Check sheet for the modelled part. Datum: model origin and axes. Units: mm. Coordinates: 2 decimals unless noted, no trailing zeros. Loops run counter-clockwise (first coordinate to the right, second up) from the corner with the lowest first, then second, coordinate; pieces in that order, holes last. Notation, with made-up numbers: M 54,29 L 103,29 A19 cw 103,56 Z; hole C 54,-9.5 d2. An arc over 180 degrees is marked long. Use CSV: the item, a comma, the result in double quotes. Start each with the question number.
(1) Section check C-C on y = 1. Record the cut outline in (x, z), and give its area (3 significant figures).
(2) Go/stop test with flat-tipped pins: pin 1 Ø2 at (y, z) = (6.5, 11) entering from -X; pin 2 Ø4 at (x, y) = (-10, 3.5) entering from -Z. Record where each tip stops, or that it passes through.
(3) Section check D-D on y = 9.25. Record the cut outline in (x, z), and give its area (3 significant figures).
(4) Scan lines: line 1 (X direction, y = -0.5, z = 6); line 2 (X direction, y = 0.5, z = 11.25); line 3 (X direction, y = -11.75, z = 18.25). Record each from-to range of solid material in increasing order.
(5) Section check A-A on z = 14. Record the cut outline in (x, y), and give its area (3 significant figures).
(6) Section check B-B on y = -2.5. Record the cut outline in (x, z).
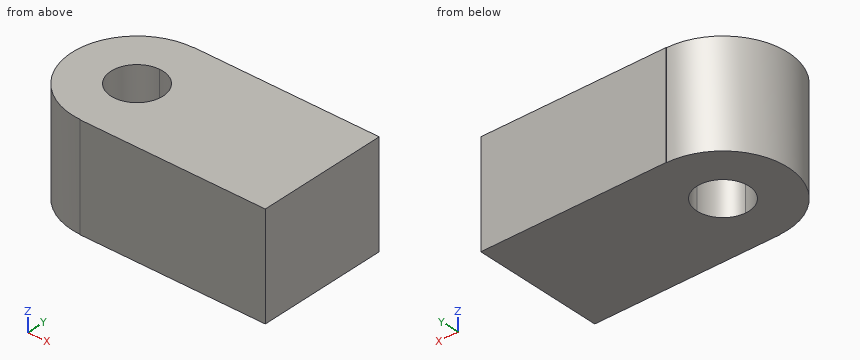
from build123d import *

# Parameters (mm, degrees)
F1_DEPTH = 20


with BuildPart() as f1:
    # F0 (on Top) → F1 (new body)
    with BuildSketch(Plane.XY):
        with BuildLine():
            Line((-12.4044854931, 4.3749214336), (-12.4044854931, 11.8749214336))
            ThreePointArc((-12.4044854931, 11.8749214336), (-24.9044854931, -0.6250785664), (-12.4044854931, -13.1250785664))
            Line((-12.4044854931, -13.1250785664), (-12.4044854931, -5.6250785664))
            ThreePointArc((-12.4044854931, -5.6250785664), (-17.4044854931, -0.6250785664), (-12.4044854931, 4.3749214336))
        make_face()
        with BuildLine():
            ThreePointArc((0.0955145069, -0.6250785664), (-3.5656507283, 8.2137561985), (-12.4044854931, 11.8749214336))
            Line((-12.4044854931, 11.8749214336), (-12.4044854931, 4.3749214336))
            ThreePointArc((-12.4044854931, 4.3749214336), (-8.8689515872, 2.9104553396), (-7.4044854931, -0.6250785664))
            ThreePointArc((-7.4044854931, -0.6250785664), (-8.8689515872, -4.1606124723), (-12.4044854931, -5.6250785664))
            Line((-12.4044854931, -5.6250785664), (-12.4044854931, -13.1250785664))
            ThreePointArc((-12.4044854931, -13.1250785664), (-3.5656507283, -9.4639133312), (0.0955145069, -0.6250785664))
        make_face()
        with BuildLine():
            Line((23.2241750516, 11.9398952645), (-12.4044854931, 11.9398952645))
            Line((-12.4044854931, 11.9398952645), (-12.4044854931, 11.8749214336))
            ThreePointArc((-12.4044854931, 11.8749214336), (-3.5656507283, 8.2137561985), (0.0955145069, -0.6250785664))
            ThreePointArc((0.0955145069, -0.6250785664), (-3.5656507283, -9.4639133312), (-12.4044854931, -13.1250785664))
            Line((-12.4044854931, -13.1250785664), (-12.4044854931, -13.1900523973))
            Line((-12.4044854931, -13.1900523973), (23.2241750516, -13.1900523973))
            Line((23.2241750516, -13.1900523973), (23.2241750516, 11.9398952645))
        make_face()
    extrude(amount=F1_DEPTH)


solid = f1.part
Outcome:
1,outline,"M -24.8,0 L -17.13,0 L -17.13,20 L -24.8,20 Z; M -7.68,0 L 23.22,0 L 23.22,20 L -7.68,20 Z"
1,area,"771 mm²"
2,pin 1,"stops at x = -23.3"
2,pin 2,"stops at z = 0"
3,outline,"M -20.07,0 L 23.22,0 L 23.22,20 L -20.07,20 Z"
3,area,"866 mm²"
4,line 1,"x = -24.9 to -17.4, -7.41 to 23.22"
4,line 2,"x = -24.85 to -17.28, -7.53 to 23.22"
4,line 3,"x = -18.1 to 23.22"
5,outline,"M -12.4,-13.19 L 23.22,-13.19 L 23.22,11.94 L -12.4,11.94 L -12.4,11.87 A12.5 ccw -12.4,-13.13 Z; hole C -12.4,-0.63 d10"
5,area,"1,060 mm²"
6,outline,"M -24.76,0 L -17.04,0 L -17.04,20 L -24.76,20 Z; M -7.77,0 L 23.22,0 L 23.22,20 L -7.77,20 Z"
